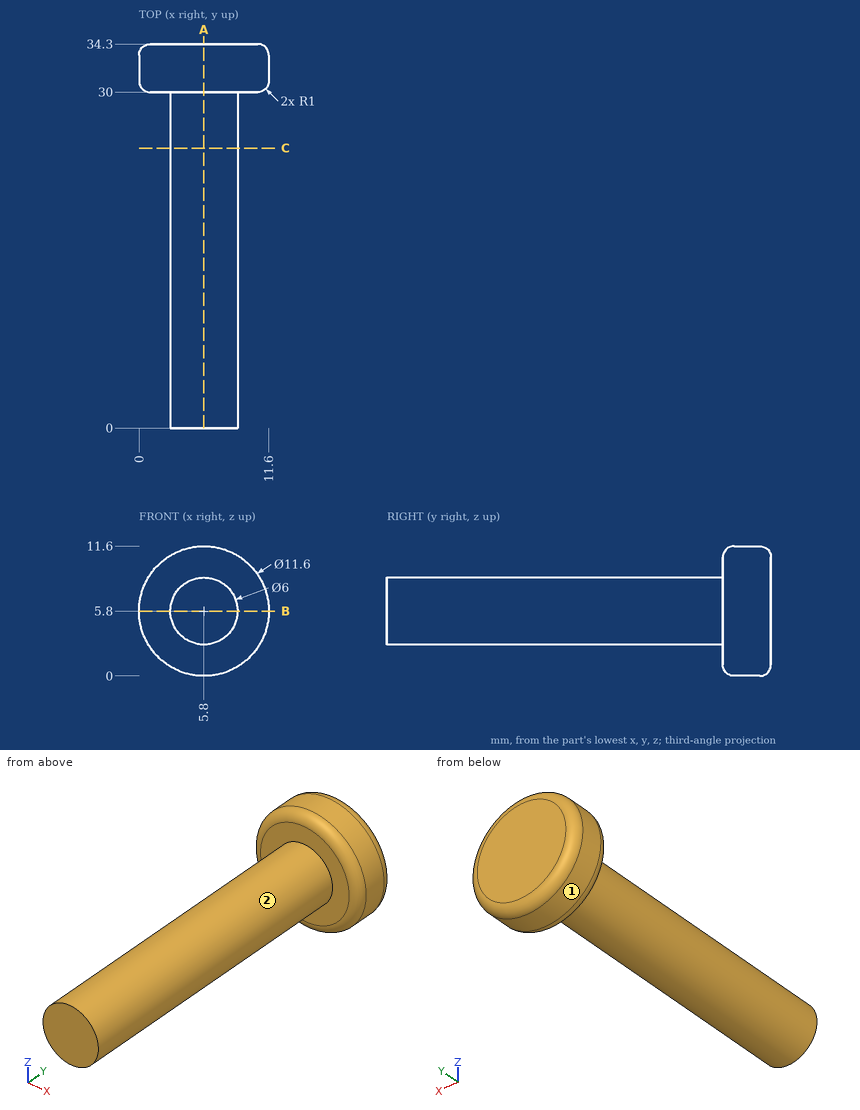
Study the drawing (mm; zero at the part's minimum x, y, z) and answer. A direction names the side the tool comes from. Coordinates: 2 decimals unless noted, no trailing zeros. Write each loop counter-clockwise with the first axis right and the second up, starting at its lowest first coordinate (ties: lowest second). Pieces come first, ordered by that corner, then holes. Notation, with made-up numbers: (67.5, -16) - (83.5, -16) arc R24 cw to (83.5, -6) - close; hole circle Ø1 at (-36.5, 32). An arc over 180 degrees is marked (long way). One line per question, with ' | ' between items.
1) For the marked faces 1 and 2, determine the directions among +Z, -Z, +X, -X, +Y, -Y from which every point of the face is accessible in a straight line to the end or side of a thin tool.
Checks:
face 1: +Y, -Y | face 2: -Y
2) Find section A-A, the plane x = 5.8. Determine the outline of the cut face in (y, z).
Checks:
outline: (0, 2.8) - (30, 2.8) - (30, 1) arc R1 ccw to (31, 0) - (33.3, 0) arc R1 ccw to (34.3, 1) - (34.3, 10.6) arc R1 ccw to (33.3, 11.6) - (31, 11.6) arc R1 ccw to (30, 10.6) - (30, 8.8) - (0, 8.8) - close
3) Find section B-B, the plane z = 5.8. Determine the outline of the cut face in (x, y), and give its area (3 significant figures).
Checks:
outline: (0, 31) arc R1 ccw to (1, 30) - (2.8, 30) - (2.8, 0) - (8.8, 0) - (8.8, 30) - (10.6, 30) arc R1 ccw to (11.6, 31) - (11.6, 33.3) arc R1 ccw to (10.6, 34.3) - (1, 34.3) arc R1 ccw to (0, 33.3) - close | area: 229 mm2
4) Find section C-C, the plane y = 25. Determine the outline of the cut face in (x, z), and give its area (3 significant figures).
Checks:
outline: circle Ø6 at (5.8, 5.8) | area: 28.3 mm2
5) Flat-ended cylindrical pins translate along their axes: P1, Ø2, axis at y = 8.5, z = 9.5, coming from the +X side; P2, Ø3, axis at x = 8, z = 10.5, coming from the -Y side; P3, Ø2, axis at y = 17.5, z = 5, coming from the +X side. Find the tip coordinate at first contact, or state that the pin passes through.
Checks:
P1: x = 7.11 | P2: y = 30 | P3: x = 8.8
6) Consider probe 1 along Y at (x, z) = (2.75, 7.75); probe 2 along X at (y, z) = (14, 6); probe 3 along Z at (x, y) = (5.75, 14). Determine where each line is inside the solid, lowest interval first. Write a range as [from, to].
Checks:
probe 1: [30, 34.3] | probe 2: [2.81, 8.79] | probe 3: [2.8, 8.8]
